Geometry check sheet. Reference: drawing and pictorial views, mm from the part's lowest x, y, z. A direction names the side the tool comes from. Coordinates: 2 decimals unless noted, no trailing zeros. Loops run counter-clockwise (first coordinate to the right, second up) from the corner with the lowest first, then second, coordinate; pieces in that order, holes last. Notation, with made-up numbers: (52.25, -25.75) -> (95.25, -25.75) arc R7 ccw to (95.25, -13.75) -> close; hole circle Ø7 at (40, 76.5). An arc over 180 degrees is marked (long way). Answer as a JSON object with one key per item and string values.
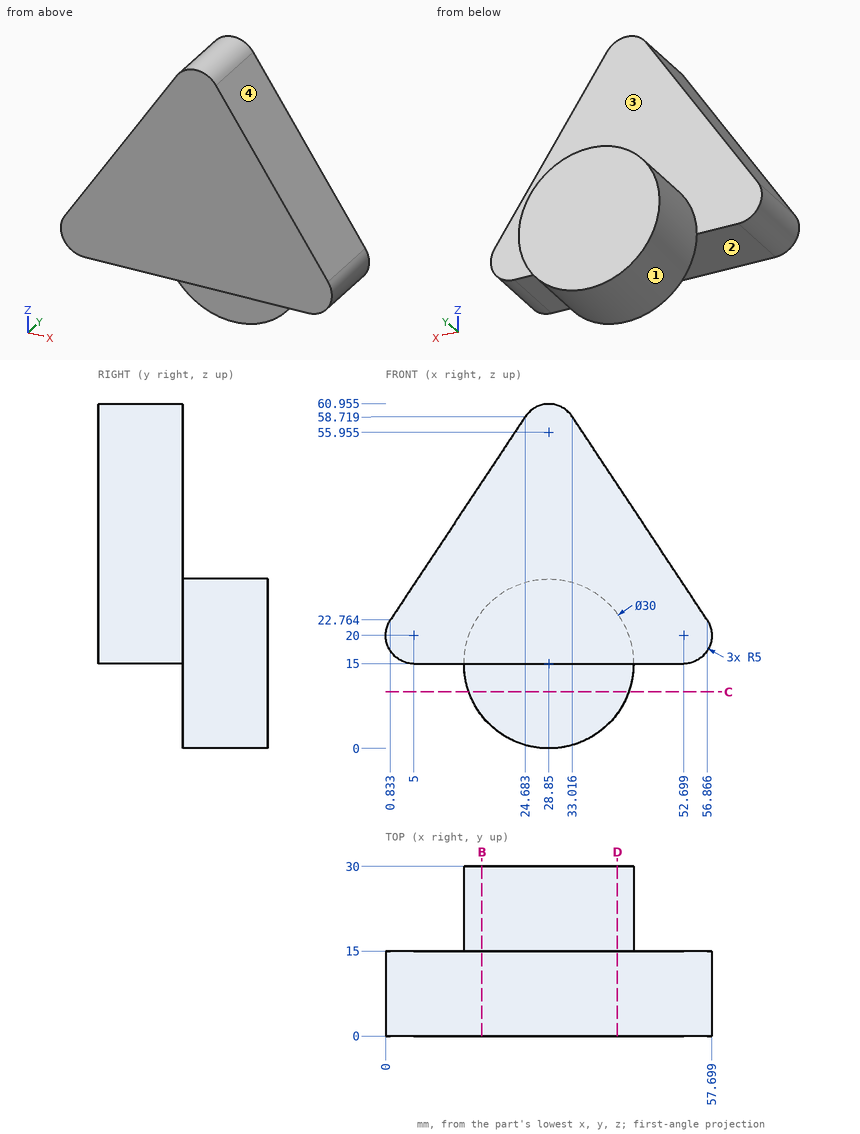
1. Depth check by flat-ended pin: P1, Ø1.5, axis at x = 11.5, z = 32, coming from the +Y side; P2, Ø12, axis at x = 44.5, y = 12, coming from the +Z side; P3, Ø6, axis at y = 16, z = 24, coming from the +X side. Enter the tip coordinate at first touch or a pass-through.
Evaluation:
{"P1": "stops at y = 15", "P2": "stops at z = 50.45", "P3": "stops at x = 57.56"}
2. Tool access check on the marked faces 1, 2, 3 and 4. Record the directions out of +Z, -Z, +X, -X, +Y, -Y that give a thin tool (end or side, any length) a straight path to the whole face; none if there is none.
Evaluation:
{"face 1": "+Y", "face 2": "-Z, +X, -X, -Y", "face 3": "+Z, +Y", "face 4": "+Z, +X, +Y, -Y"}
3. Section check C-C, the plane z = 10. Record the boundary of the cut face in (x, y).
Evaluation:
{"outline": "(14.71, 15) -> (42.99, 15) -> (42.99, 30) -> (14.71, 30) -> close"}
4. Section check B-B, the plane x = 17. Record the boundary of the cut face in (y, z).
Evaluation:
{"outline": "(0, 15) -> (15, 15) -> (15, 5.8) -> (30, 5.8) -> (30, 24.2) -> (15, 24.2) -> (15, 47.14) -> (0, 47.14) -> close"}
5. Section check D-D, the plane x = 41. Record the boundary of the cut face in (y, z) (1 decimal).
Evaluation:
{"outline": "(0, 15) -> (15, 15) -> (15, 6.2) -> (30, 6.2) -> (30, 23.8) -> (15, 23.8) -> (15, 46.7) -> (0, 46.7) -> close"}
6. Thickness scan on probe 1 along Y at (x, z) = (23.5, 56.5); probe 2 along Y at (x, z) = (37, 4); probe 3 along Z at (x, y) = (40, 14.5). Record the ranges inside material, lowest first. Write a range as from..to.
Evaluation:
{"probe 1": "y = 0..15", "probe 2": "y = 15..30", "probe 3": "z = 15..48.19"}
